from build123d import *

# Parameters (mm, degrees)
F1_DEPTH = 70
F3_DEPTH = 15


with BuildPart() as f1:
    # F0 (on Front) → F1 (new body, symmetric)
    with BuildSketch(Plane.XZ):
        Polygon((450, 1800), (-450, 1800), (-450, 0), (-405, 0), (-405, 1755), (405, 1755), (405, 0), (450, 0), align=None)
    extrude(amount=F1_DEPTH, both=True)

    # F2 (on Front) → F3 (join, symmetric)
    with BuildSketch(Plane.XZ):
        Polygon((405, 1755), (-405, 1755), (-405, 0), (-395, 0), (-395, 1745), (395, 1745), (395, 0), (405, 0), align=None)
    extrude(amount=F3_DEPTH, both=True)


solid = f1.part
Model file for the job. Use its own axes, mm. A direction names the side the tool comes from. Give positions to 0.01 mm unless a question says otherwise; leave off trailing zeros. Order: outer loops, then holes, each group sorted by start corner. A loop starts at its lowest first (then second) coordinate and runs counter-clockwise, first axis right, second up. Notation, with made-up numbers: (-21.75, 40.5) - (-16.75, 40.5) arc R18 ccw to (-16.75, 53.5) - close; hole circle Ø8 at (-7, -20). An arc over 180 degrees is marked (long way). Write item = value, one per line. Start each with the question number.
1. Cut at A-A, the plane z = 1327. List the corners of the cut face in (x, y).
2. Drop a flat-ended pin along its axis: P1, Ø9, axis at x = -160.5, y = -1.5, coming from the -Z side. Give the stop position or say it passes through.
3. Two-plate mould, pull along X, no slides. Class faces 1 (the flat face through (-429, -1, 0)), 2 (the flat face through (-450, -1, 913)), 3 (the flat face through (-6, -43, 1755)): pulls with the +X half, pulls with the -X half, needs draft (parallel to the pull), parting line crosses it, or undercut.
4. Cut at B-B, the plane y = 41. List the corners of the cut face in (x, z).
5. Probe line 1 along X through (y, z) = (-16.5, 493); line 2 along X through (y, z) = (0.5, 928); line 3 along Z through (x, y) = (-91, -39). List the from-to ranges inside material, lowest first.
6. Cut at C-C, the plane x = -154. List the corners of the cut face in (y, z).
7. Which spindle directions (+Z, -Z, +X, -X, +Y, -Y) get a long thin tool onto all of the face, cutting with end or side? Do faces 4 (the flat face through (450, -1, 887)), 5 (the flat face through (-405, 42, 865)), 6 (the flat face through (-405, -43, 865)). Say none if no direction does.
Taken from the geometry:
q1.outline = (-450, -70) - (-405, -70) - (-405, -15) - (-395, -15) - (-395, 15) - (-405, 15) - (-405, 70) - (-450, 70) - close; (395, -15) - (405, -15) - (405, -70) - (450, -70) - (450, 70) - (405, 70) - (405, 15) - (395, 15) - close
q2.P1 = 1745
q3.face_1 = needs draft
q3.face_2 = pulls with the -X half
q3.face_3 = undercut
q4.outline = (-450, 0) - (-405, 0) - (-405, 1755) - (405, 1755) - (405, 0) - (450, 0) - (450, 1800) - (-450, 1800) - close
q5.line_1 = -450 to -405, 405 to 450
q5.line_2 = -450 to -395, 395 to 450
q5.line_3 = 1755 to 1800
q6.outline = (-70, 1755) - (-15, 1755) - (-15, 1745) - (15, 1745) - (15, 1755) - (70, 1755) - (70, 1800) - (-70, 1800) - close
q7.face_4 = +Z, -Z, +X, +Y, -Y
q7.face_5 = -Z, +Y
q7.face_6 = -Z, -Y
